```python
from build123d import *

# Parameters (mm, degrees)
SKETCH1_R                   = 76.1
BOSS_EXTRUDE1_DEPTH         = 3.175
SKETCH3_W                   = 15.4
SKETCH3_H                   = 3.175
CUT_EXTRUDE1_DEPTH          = 108.66847554
SKETCH4_R                   = 0.5
CUT_EXTRUDE2_DEPTH          = 108.66847554
SKETCH_PATTERN1_DEPTH       = 3.175
CIRPATTERN1_COUNT           = 4
CIRPATTERN1_COPY_1_SKETCH_R = 0.5
CIRPATTERN1_COPY_1_DEPTH    = 108.66847554
CIRPATTERN1_COPY_2_SKETCH_R = 0.5
CIRPATTERN1_COPY_2_DEPTH    = 108.66847554
CIRPATTERN1_COPY_3_SKETCH_R = 0.5
CIRPATTERN1_COPY_3_DEPTH    = 108.66847554
CIRPATTERN1_COPY_4_DEPTH    = 3.175
CIRPATTERN1_COPY_5_DEPTH    = 3.175
CIRPATTERN1_COPY_6_DEPTH    = 3.175


# Read off the part's stored shape, not the designer's step: Sketch-Pattern1
with BuildPart() as part:
    # Sketch1 → Boss-Extrude1 (new body)
    with BuildSketch(Plane(origin=(0, 0, 0), x_dir=(1, 0, 0), z_dir=(0, 1, 0))):
        with Locations(Location((0, 0, 0), (0, 0, 270))):
            Circle(SKETCH1_R)
    extrude(amount=BOSS_EXTRUDE1_DEPTH)

    # Sketch3 → Cut-Extrude1 (cut, symmetric)
    with BuildSketch(Plane(origin=(0, 3.175, 0), x_dir=(1, 0, 0), z_dir=(0, 1, 0))):
        with Locations((-17.7, 58.6875)):
            Rectangle(SKETCH3_W, SKETCH3_H)
        with Locations((17.7, 58.6875)):
            Rectangle(SKETCH3_W, SKETCH3_H)
    cut_extrude1 = extrude(amount=CUT_EXTRUDE1_DEPTH, both=True, mode=Mode.SUBTRACT)

    # Sketch4 → Cut-Extrude2 (cut, symmetric)
    with BuildSketch(Plane(origin=(0, 3.175, 0), x_dir=(1, 0, 0), z_dir=(0, 1, 0))):
        with Locations((-25.046446609, 59.921446609)):
            Circle(SKETCH4_R)
        with Locations((-25.046446609, 57.453553391)):
            Circle(SKETCH4_R)
    cut_extrude2 = extrude(amount=CUT_EXTRUDE2_DEPTH, both=True, mode=Mode.SUBTRACT)

    # Sketch-Pattern1 outline → Sketch-Pattern1 (cut)
    with BuildSketch(Plane(origin=(0, 0, 0), x_dir=(1, 0, 0), z_dir=(0, 1, 0))):
        with BuildLine():
            Line((10, 60.275), (10.707106781, 60.275))
            ThreePointArc((10.707106781, 60.275), (10.353553391, 60.421446609), (10, 60.275))
        make_face()
        with BuildLine():
            Line((10.707106781, 57.1), (10, 57.1))
            ThreePointArc((10, 57.1), (10.353553391, 56.953553391), (10.707106781, 57.1))
        make_face()
        with BuildLine():
            Line((10, 57.1), (10, 57.807106781))
            ThreePointArc((10, 57.807106781), (9.853553391, 57.453553391), (10, 57.1))
        make_face()
        with BuildLine():
            Line((10, 59.567893219), (10, 60.275))
            ThreePointArc((10, 60.275), (9.853553391, 59.921446609), (10, 59.567893219))
        make_face()
    sketch_pattern1 = extrude(amount=SKETCH_PATTERN1_DEPTH, mode=Mode.SUBTRACT)

    # Mirror1: Cut-Extrude2, Sketch-Pattern1 across plane
    add(cut_extrude2.mirror(Plane(origin=(0, 0, 0), x_dir=(0, 0, 1), z_dir=(1, 0, 0))), mode=Mode.SUBTRACT)
    add(sketch_pattern1.mirror(Plane(origin=(0, 0, 0), x_dir=(0, 0, 1), z_dir=(1, 0, 0))), mode=Mode.SUBTRACT)

    # CirPattern1: Cut-Extrude1, Cut-Extrude2, Sketch-Pattern1 ×4 about axis
    cirpattern1_axis = Axis((0, 0, 0), (0, 1, 0))
    add([cut_extrude1.rotate(cirpattern1_axis, i * 360 / CIRPATTERN1_COUNT) for i in range(1, CIRPATTERN1_COUNT)], mode=Mode.SUBTRACT)
    add([cut_extrude2.rotate(cirpattern1_axis, i * 360 / CIRPATTERN1_COUNT) for i in range(1, CIRPATTERN1_COUNT)], mode=Mode.SUBTRACT)
    add([sketch_pattern1.rotate(cirpattern1_axis, i * 360 / CIRPATTERN1_COUNT) for i in range(1, CIRPATTERN1_COUNT)], mode=Mode.SUBTRACT)

    # CirPattern1 copy 1 sketch → CirPattern1 copy 1 (cut, symmetric)
    with BuildSketch(Plane.ZX.offset(3.175)):
        with Locations((-25.046446609, -59.921446609)):
            Circle(CIRPATTERN1_COPY_1_SKETCH_R)
        with Locations((-25.046446609, -57.453553391)):
            Circle(CIRPATTERN1_COPY_1_SKETCH_R)
    extrude(amount=CIRPATTERN1_COPY_1_DEPTH, both=True, mode=Mode.SUBTRACT)

    # CirPattern1 copy 2 sketch → CirPattern1 copy 2 (cut, symmetric)
    with BuildSketch(Plane(origin=(0, 3.175, 0), x_dir=(1, 0, 0), z_dir=(0, 1, 0))):
        with Locations((-25.046446609, -59.921446609)):
            Circle(CIRPATTERN1_COPY_2_SKETCH_R)
        with Locations((-25.046446609, -57.453553391)):
            Circle(CIRPATTERN1_COPY_2_SKETCH_R)
    extrude(amount=CIRPATTERN1_COPY_2_DEPTH, both=True, mode=Mode.SUBTRACT)

    # CirPattern1 copy 3 sketch → CirPattern1 copy 3 (cut, symmetric)
    with BuildSketch(Plane(origin=(0, 3.175, 0), x_dir=(0, 0, -1), z_dir=(0, 1, 0))):
        with Locations((-25.046446609, -59.921446609)):
            Circle(CIRPATTERN1_COPY_3_SKETCH_R)
        with Locations((-25.046446609, -57.453553391)):
            Circle(CIRPATTERN1_COPY_3_SKETCH_R)
    extrude(amount=CIRPATTERN1_COPY_3_DEPTH, both=True, mode=Mode.SUBTRACT)

    # CirPattern1 copy 4 sketch → CirPattern1 copy 4 (cut)
    with BuildSketch(Plane.ZX):
        with BuildLine():
            Line((10, -60.275), (10.707106781, -60.275))
            ThreePointArc((10.707106781, -60.275), (10.353553391, -60.421446609), (10, -60.275))
        make_face()
        with BuildLine():
            Line((10.707106781, -57.1), (10, -57.1))
            ThreePointArc((10, -57.1), (10.353553391, -56.953553391), (10.707106781, -57.1))
        make_face()
        with BuildLine():
            Line((10, -57.1), (10, -57.807106781))
            ThreePointArc((10, -57.807106781), (9.853553391, -57.453553391), (10, -57.1))
        make_face()
        with BuildLine():
            Line((10, -59.567893219), (10, -60.275))
            ThreePointArc((10, -60.275), (9.853553391, -59.921446609), (10, -59.567893219))
        make_face()
    extrude(amount=CIRPATTERN1_COPY_4_DEPTH, mode=Mode.SUBTRACT)

    # CirPattern1 copy 5 sketch → CirPattern1 copy 5 (cut)
    with BuildSketch(Plane(origin=(0, 0, 0), x_dir=(1, 0, 0), z_dir=(0, 1, 0))):
        with BuildLine():
            Line((10, -60.275), (10.707106781, -60.275))
            ThreePointArc((10.707106781, -60.275), (10.353553391, -60.421446609), (10, -60.275))
        make_face()
        with BuildLine():
            Line((10.707106781, -57.1), (10, -57.1))
            ThreePointArc((10, -57.1), (10.353553391, -56.953553391), (10.707106781, -57.1))
        make_face()
        with BuildLine():
            Line((10, -57.1), (10, -57.807106781))
            ThreePointArc((10, -57.807106781), (9.853553391, -57.453553391), (10, -57.1))
        make_face()
        with BuildLine():
            Line((10, -59.567893219), (10, -60.275))
            ThreePointArc((10, -60.275), (9.853553391, -59.921446609), (10, -59.567893219))
        make_face()
    extrude(amount=CIRPATTERN1_COPY_5_DEPTH, mode=Mode.SUBTRACT)

    # CirPattern1 copy 6 sketch → CirPattern1 copy 6 (cut)
    with BuildSketch(Plane(origin=(0, 0, 0), x_dir=(0, 0, -1), z_dir=(0, 1, 0))):
        with BuildLine():
            Line((10, -60.275), (10.707106781, -60.275))
            ThreePointArc((10.707106781, -60.275), (10.353553391, -60.421446609), (10, -60.275))
        make_face()
        with BuildLine():
            Line((10.707106781, -57.1), (10, -57.1))
            ThreePointArc((10, -57.1), (10.353553391, -56.953553391), (10.707106781, -57.1))
        make_face()
        with BuildLine():
            Line((10, -57.1), (10, -57.807106781))
            ThreePointArc((10, -57.807106781), (9.853553391, -57.453553391), (10, -57.1))
        make_face()
        with BuildLine():
            Line((10, -59.567893219), (10, -60.275))
            ThreePointArc((10, -60.275), (9.853553391, -59.921446609), (10, -59.567893219))
        make_face()
    extrude(amount=CIRPATTERN1_COPY_6_DEPTH, mode=Mode.SUBTRACT)


solid = part.part
```
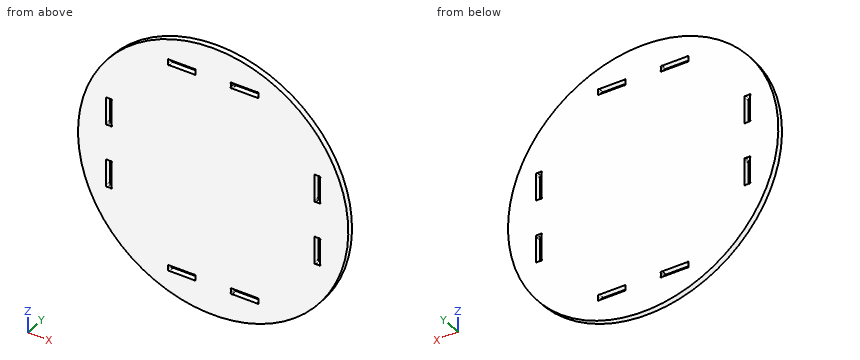
Geometry: final body of the model. Coordinates: model frame, mm. Give positions to 0.01 mm unless a question says otherwise; leave off trailing zeros. Write each loop counter-clockwise with the first axis right and the second up, starting at its lowest first coordinate (ties: lowest second). Pieces come first, ordered by that corner, then holes.
1. Section query B-B, the plane z = -42.5. Return loops of the section in (x, y) (3 decimals), then the cut area to 3 significant figures.
2. Section query C-C, the plane z = 46.5. Return loops of the section in (x, y) (3 decimals), then the cut area to 3 significant figures.
3. Pin query (flat end, axial travel): P1, Ø0.5, axis at x = -58.5, y = 1.5, coming from the -Z side; P2, Ø0.9, axis at y = 1.5, z = 59, coming from the -X side; P3, Ø1.9, axis at y = 1.5, z = 59, coming from the +X side. Return the tip coordinate at first contact, or that it passes through.
4. Line query: probe 1 along X at (y, z) = (1.7, 12.5) (3 decimals); probe 2 along X at (y, z) = (0.95, -16.5) (3 decimals); probe 3 along Z at (x, y) = (58, 0.55). Output: solid intervals per line, ascending.
5. Section query A-A, the plane y = 2.4. Count the separate pieces of the cut face and the enclosed holes in it, then the cut area to 3 significant figures.
Computed:
1. outline: (-63.127, 0) - (63.127, 0) - (63.127, 3.175) - (-63.127, 3.175) - close
1. area: 401 mm2
2. outline: (-60.241, 0) - (60.241, 0) - (60.241, 3.175) - (-60.241, 3.175) - close
2. area: 383 mm2
3. P1: stops at z = -48.97
3. P2: stops at x = -48.61
3. P3: stops at x = 49.21
4. probe 1: x = -75.066 to -60.275, -57.1 to 57.1, 60.275 to 75.066
4. probe 2: x = -74.29 to -60.275, -57.1 to 57.1, 60.275 to 74.29
4. probe 3: z = -49.27 to -25.4, -10 to 10, 25.4 to 49.27
5. separate pieces: 1
5. enclosed holes: 8
5. area: 17,800 mm2
